from build123d import *

# Parameters (mm, degrees)
SKETCH1_R           = 4.25
BASEHEAD_DEPTH      = 5
SKETCH2_R           = 2.5
BASEBODY_DEPTH      = 25
HEXAGONSOCKET_DEPTH = 2.5
TOPFILLET_R         = 0.2
CHAMFER1_SIZE       = 0.1


with BuildPart() as part:
    # Sketch1 → BaseHead (new body)
    with BuildSketch(Plane(origin=(0, 0, 0), x_dir=(0, 0, -1), z_dir=(1, 0, 0))):
        Circle(SKETCH1_R)
    extrude(amount=BASEHEAD_DEPTH)

    # Sketch2 → BaseBody (add)
    with BuildSketch(Plane(origin=(5, 0, 0), x_dir=(0, 0, -1), z_dir=(1, 0, 0))):
        Circle(SKETCH2_R)
    extrude(amount=BASEBODY_DEPTH)

    # Sketch3 → HexagonSocket (cut)
    with BuildSketch(Plane(origin=(0, 0, 0), x_dir=(0, 0, -1), z_dir=(1, 0, 0))):
        Polygon((2.309401077, 0), (1.154700538, 2), (-1.154700538, 2), (-2.309401077, 0), (-1.154700538, -2), (1.154700538, -2), align=None)
    extrude(amount=HEXAGONSOCKET_DEPTH, mode=Mode.SUBTRACT)

    # Sketch4 → Cut-Revolve1 (revolve, cut)
    with BuildSketch(Plane(origin=(-4.19613823, 0.75, 0), x_dir=(-1, 0, 0), z_dir=(0, 0, 1))):
        Polygon((-6.69613823, 2.75), (-7.850838768, 0.75), (-6.69613823, 0.75), align=None)
    revolve(axis=Axis((0.838992387, 0, 0), (-1, 0, 0)), mode=Mode.SUBTRACT)

    # TopFillet
    topfillet_edges = [part.edges().sort_by_distance(p)[0] for p in [
        (0, 0, 4.25),
    ]]
    fillet(topfillet_edges, radius=TOPFILLET_R)

    # Chamfer1
    chamfer1_edges = [part.edges().sort_by_distance(p)[0] for p in [
        (30, 0, 2.5),
    ]]
    chamfer(chamfer1_edges, length=CHAMFER1_SIZE)


solid = part.part
CAD build for the part. Positions are in the model's coordinates, mm. A direction names the side the tool comes from. Coordinates: 2 decimals unless noted, no trailing zeros. Order: outer loops, then holes, each group sorted by start corner. A loop starts at its lowest first (then second) coordinate and runs counter-clockwise, first axis right, second up. Notation, with made-up numbers: (-5, -22) -> (15, -22) arc R11 cw to (15, -3) -> close; hole circle Ø2 at (87.25, 86). An arc over 180 degrees is marked (long way). Answer in a Markdown table with one row per item.
1) Drill centre lines: line 1 (X direction, y = 2.25, z = -1.25); line 2 (Y direction, x = 13.75, z = 0); line 3 (Z direction, x = 1.75, y = 3.75). Where is each one in solid material? Low to high.
Check values:
| item | result |
|---|---|
| line 1 | 0 to 5 |
| line 2 | -2.5 to 2.5 |
| line 3 | -2 to 2 |
2) Band-saw the part on A-A (x = 17.25). List the corners of the cut face in (y, z), and give its area (3 significant figures).
Check values:
| item | result |
|---|---|
| outline | circle Ø5 at (0, 0) |
| area | 19.6 mm2 |
3) Mould opens along Y. For faces 1 (the face through (1, -2, 0)), 2 (the face through (5, -2, -2)), 3 (the face through (17.28, -2.44, 0.54)) say: pulls with the +Y half, pulls with the -Y half, needs draft (parallel to the pull), parting line crosses it, or undercut.
Check values:
| item | result |
|---|---|
| face 1 | undercut |
| face 2 | needs draft |
| face 3 | parting line crosses it |
4) Which spindle directions (+Z, -Z, +X, -X, +Y, -Y) get a long thin tool onto all of the face, cutting with end or side? Do faces 4 (the face through (0, -1, 2)), 5 (the face through (1, 2, 0)). Say none if no direction does.
Check values:
| item | result |
|---|---|
| face 4 | +Z, -Z, -X, +Y, -Y |
| face 5 | -X |
5) Flat gauge pins, fed straight in: P1, Ø4, axis at x = 19, y = -3.5, coming from the +Z side; P2, Ø1.5, axis at y = 0.5, z = -0.5, coming from the -X side; P3, Ø0.5, axis at y = -1.5, z = 1, coming from the -X side. Where does each tip first touch, or does it go through?
Check values:
| item | result |
|---|---|
| P1 | z = 2 |
| P2 | x = 2.81 |
| P3 | x = 2.5 |
